Input: part model. Units: mm. Frame: model coordinates. A direction names the side the tool comes from. Round coordinates to 2 decimals unless told otherwise and drop trailing zeros. Loops run counter-clockwise (first coordinate to the right, second up) from the corner with the lowest first, then second, coordinate; pieces in that order, holes last. Notation, with made-up numbers: (86, 21.25) -> (138, 21.25) arc R24 ccw to (138, 52.25) -> close; hole circle Ø10 at (-1, -7.5). An arc over 180 degrees is marked (long way). Answer as a JSON object with one key per item and string values. Group by question number.
Item 1: Pin query (flat end, axial travel): pin 1 (1.6 mm diameter, centred on x = 3.5, y = 9, fed in from +Z); pin 2 (7 mm diameter, centred on y = 10.5, z = 8.5, fed in from +X); pin 3 (3.5 mm diameter, centred on y = 10, z = 10, fed in from -X). Return the tip coordinate at first contact, or that it passes through.
Item 2: Draft query along Z for faces 6 (the flat face through (4, 8, 7.25)), 7 (the cylindrical face through (-1.4, 2.54, 18.64)), 8 (the flat face through (-1.1, 17, -6.1)). Return one class per face: released by +Z, released by -Z, zero draft, split by the parting line, or undercut.
Item 3: Section query C-C on x = -1.5. Return loops of the section in (y, z).
Item 4: Set-up query: faces 1 (the flat face through (0.5, 6, 9)), 2 (the flat face through (-4.5, 10, 9)), 3 (the flat face through (3, 9, 11)), 4 (the cylindrical face through (1.732, 9.421, 10.095)), 5 (the flat face through (4.5, 6, 9)). Return all of +Z, -Z, +X, -X, +Y, -Y with unobstructed straight access to the full face (end or side cutting, diameter ignored); none if empty.
Item 5: Material intervals for line 1 (Z direction, x = 2.1, y = 8.5); line 2 (X direction, y = 11, z = 0); line 3 (X direction, y = 12.75, z = 9), sorted ascending. Write a range as [from, to].
Item 6: Section query D-D on x = -4. Return loops of the section in (y, z).
Item 7: Section query B-B on y = 2.25. Return loops of the section in (x, z), and give its area (3 significant figures).
Item 8: Section query A-A on z = 12. Return loops of the section in (x, y).
from build123d import *

# Parameters (mm, degrees)
SKETCH_1_R                  = 7.5
SKETCH_1_R_2                = 6
EXTRUDE_1_DEPTH             = 17
CUT_EXTRUDE_1_REACH         = 25.88
CUT_EXTRUDE_1_END_RADIUS    = 6
SKETCH_2_W                  = 1
SKETCH_2_H                  = 17
SKETCH_3_W                  = 4
SKETCH_3_H                  = 17
EXTRUDE_2_DEPTH             = 5
EXTRUDE_2_DIRECTION_2_REACH = 25.88
CUT_EXTRUDE_START           = -2
CUT_EXTRUDE_4_DEPTH         = 2
CUT_EXTRUDE_2_REACH         = 26.274
SKETCH_4_R                  = 1.25
CUT_EXTRUDE_3_DEPTH         = 1.5
EXTRUDE_3_DEPTH             = 5
CUT_EXTRUDE_5_REACH         = 26.094
SKETCH_9_R                  = 1.35
FILLET_1_R                  = 3


with BuildPart() as part:
    # 草图1 → 凸台-拉伸1 (new body)
    with BuildSketch(Plane(origin=(0, 0, 0), x_dir=(1, 0, 0), z_dir=(0, 1, 0))):
        with Locations(Location((0, 0, 0), (0, 0, 270))):
            Circle(SKETCH_1_R)
        with Locations(Location((0, 0, 0), (0, 0, 270))):
            Circle(SKETCH_1_R_2, mode=Mode.SUBTRACT)
    extrude(amount=EXTRUDE_1_DEPTH)

    # 切除-拉伸1: up to this cylinder (the profile starts outside it)
    cut_extrude_1_end = Plane(origin=(0, 8.5, 0), z_dir=(0, -1, 0)) * Cylinder(CUT_EXTRUDE_1_END_RADIUS, 64.76, mode=Mode.PRIVATE)
    # 草图2 → 切除-拉伸1 (cut, up to the surface)
    with BuildSketch(Plane.XY.offset(7.5), mode=Mode.PRIVATE) as cut_extrude_1_sk1:
        with Locations((0, 8.5)):
            Rectangle(SKETCH_2_W, SKETCH_2_H)
    cut_extrude_1_tool1 = extrude(cut_extrude_1_sk1.sketch, amount=-CUT_EXTRUDE_1_REACH, mode=Mode.PRIVATE) - cut_extrude_1_end
    add(cut_extrude_1_tool1.solids().sort_by_distance((0, 8.5, 7.5))[0], mode=Mode.SUBTRACT)

    # 草图3 → 凸台-拉伸2 (add)
    with BuildSketch(Plane.XY.offset(7.5)):
        with Locations((-2.5, 8.5)):
            Rectangle(SKETCH_3_W, SKETCH_3_H)
        with Locations((2.5, 8.5)):
            Rectangle(SKETCH_3_W, SKETCH_3_H)
    extrude(amount=EXTRUDE_2_DEPTH)

    # 草图3 → 凸台-拉伸2 direction 2 (add, up to next)
    with BuildSketch(Plane.XY.offset(7.5), mode=Mode.PRIVATE) as extrude_2_direction_2_sk1:
        with Locations((-2.5, 8.5)):
            Rectangle(SKETCH_3_W, SKETCH_3_H)
    extrude_2_direction_2_tool1 = extrude(extrude_2_direction_2_sk1.sketch, amount=-EXTRUDE_2_DIRECTION_2_REACH, mode=Mode.PRIVATE) - part.part
    # 草图3 → 凸台-拉伸2 direction 2 (add, up to next)
    with BuildSketch(Plane.XY.offset(7.5), mode=Mode.PRIVATE) as extrude_2_direction_2_sk2:
        with Locations((2.5, 8.5)):
            Rectangle(SKETCH_3_W, SKETCH_3_H)
    extrude_2_direction_2_tool2 = extrude(extrude_2_direction_2_sk2.sketch, amount=-EXTRUDE_2_DIRECTION_2_REACH, mode=Mode.PRIVATE) - part.part
    add(extrude_2_direction_2_tool1.solids().sort_by_distance((-2.5, 8.5, 7.5))[0])
    add(extrude_2_direction_2_tool2.solids().sort_by_distance((2.5, 8.5, 7.5))[0])

    # 草图7 → 切除-拉伸4 (cut)
    with BuildSketch(Plane(origin=(0, 17, 0), x_dir=(1, 0, 0), z_dir=(0, 1, 0)).offset(CUT_EXTRUDE_START)):
        with BuildLine():
            Line((-4.5, -6), (-4.5, -12.5))
            Line((-4.5, -12.5), (4.5, -12.5))
            Line((4.5, -12.5), (4.5, -6))
            ThreePointArc((4.5, -6), (0, -7.5), (-4.5, -6))
        make_face()
    extrude(amount=CUT_EXTRUDE_4_DEPTH, mode=Mode.SUBTRACT)

    # 切除-拉伸2: up to this face of the body (flat: up to its plane)
    cut_extrude_2_end = Plane(part.part.faces().sort_by_distance((4.5, 7.5, 9.25))[0])
    # 草图4 → 切除-拉伸2 (cut, up to the picked face)
    with BuildSketch(Plane.ZY.offset(4.5), mode=Mode.PRIVATE) as cut_extrude_2_sk1:
        with Locations(Location((9.25, 8.5, 0), (0, 0, 270))):
            Circle(SKETCH_4_R)
    cut_extrude_2_tool1 = split(extrude(cut_extrude_2_sk1.sketch, amount=-CUT_EXTRUDE_2_REACH, mode=Mode.PRIVATE), bisect_by=cut_extrude_2_end, keep=Keep.BOTH, mode=Mode.PRIVATE)
    add(cut_extrude_2_tool1.solids().sort_by(Axis((-4.5, 8.5, 9.25), (1, 0, 0)))[0], mode=Mode.SUBTRACT)

    # 草图5 → 切除-拉伸3 (cut)
    with BuildSketch(Plane(origin=(4.5, 0, 0), x_dir=(0, 0, -1), z_dir=(1, 0, 0))):
        Polygon((-9.25, 6.190598923), (-7.25, 7.345299462), (-7.25, 9.654700538), (-9.25, 10.809401077), (-11.25, 9.654700538), (-11.25, 7.345299462), align=None)
    extrude(amount=-CUT_EXTRUDE_3_DEPTH, mode=Mode.SUBTRACT)

    # 草图8 → 凸台-拉伸3 (add)
    with BuildSketch(Plane(origin=(0, 0, 0), x_dir=(1, 0, 0), z_dir=(0, 1, 0))):
        Polygon((-7.5, 0), (-7.5, -19.5), (-0.5, -19.5), (-0.5, -12.5), (-4.5, -12.5), (-4.5, -6), align=None)
    extrude(amount=EXTRUDE_3_DEPTH)

    # 草图9 → 切除-拉伸5 (cut, up to next)
    with BuildSketch(Plane(origin=(0, 5, 0), x_dir=(1, 0, 0), z_dir=(0, 1, 0)), mode=Mode.PRIVATE) as cut_extrude_5_sk1:
        with Locations(Location((-4, -16, 0), (0, 0, 270))):
            Circle(SKETCH_9_R)
    cut_extrude_5_tool1 = extrude(cut_extrude_5_sk1.sketch, amount=-CUT_EXTRUDE_5_REACH, mode=Mode.PRIVATE) & part.part
    add(cut_extrude_5_tool1.solids().sort_by_distance((-4, 5, 16))[0], mode=Mode.SUBTRACT)

    # 圆角1
    fillet_1_edges = [part.edges().sort_by_distance(p)[0] for p in [
        (-7.5, 2.5, 19.5),
        (-0.5, 2.5, 19.5),
    ]]
    fillet(fillet_1_edges, radius=FILLET_1_R)


solid = part.part
Solved:
{
 "1": {"pin 1": "z = 12.5", "pin 2": "x = 5.59", "pin 3": "x = -4.5"},
 "2": {"face 6": "undercut", "face 7": "released by +Z", "face 8": "zero draft"},
 "3": {"outline": "(0, -7.35) -> (17, -7.35) -> (17, -5.81) -> (0, -5.81) -> close; (0, 5.81) -> (17, 5.81) -> (17, 7.35) -> (15, 7.35) -> (15, 12.5) -> (5, 12.5) -> (5, 18.74) -> (0, 18.74) -> close; hole circle Ø2.5 at (8.5, 9.25)"},
 "4": {"face 1": "+Z, +Y, -Y", "face 2": "+Z, -X, +Y", "face 3": "+X", "face 4": "+X, -X", "face 5": "+Z, +X, +Y, -Y"},
 "5": {"line 1": "[-7.2, -5.62], [5.62, 8], [10.5, 12.5]", "line 2": "[-7.5, -6], [6, 7.5]", "line 3": "[-4.5, -0.5], [0.5, 4.5]"},
 "6": {"outline": "(0, -6.34) -> (17, -6.34) -> (17, -4.47) -> (0, -4.47) -> close; (0, 4.47) -> (17, 4.47) -> (17, 6.34) -> (15, 6.34) -> (15, 12.5) -> (5, 12.5) -> (5, 14.65) -> (0, 14.65) -> close; (0, 17.35) -> (5, 17.35) -> (5, 19.5) -> (0, 19.5) -> close; hole circle Ø2.5 at (8.5, 9.25)"},
 "7": {"outline": "(-7.5, 0) arc R7.5 ccw (long way) to (4.5, 6) -> (4.5, 12.5) -> (0.5, 12.5) -> (0.5, 5.98) arc R6 cw (long way) to (-0.5, 5.98) -> (-0.5, 16.5) arc R3 ccw to (-3.5, 19.5) -> (-4.5, 19.5) arc R3 ccw to (-7.5, 16.5) -> close; hole circle Ø2.7 at (-4, 16)", "area": "171 mm²"},
 "8": {"outline": "(-7.5, 0) -> (-0.5, 0) -> (-0.5, 15) -> (-4.5, 15) -> (-4.5, 5) -> (-7.5, 5) -> close; (0.5, 0) -> (4.5, 0) -> (4.5, 15) -> (0.5, 15) -> close"}
}
